The listing builds one solid part. Answer for the finished solid, in the listing's coordinates (mm). Face numbers are marked on the shaded views. A direction names the side the tool comes from. Round coordinates to 2 decimals unless told otherwise and drop trailing zeros. Loops run counter-clockwise (first coordinate to the right, second up) from the corner with the lowest first, then second, coordinate; pieces in that order, holes last. Notation, with made-up numbers: (-27.5, -17) - (-11.5, -17) arc R7 ccw to (-11.5, -7) - close; hole circle Ø4 at (40.25, 38.5). An arc over 180 degrees is marked (long way). One line per item, written item: value.
Autodesk Inventor part; units mm, degrees
ref_plane "to_body_XY" through (0, 0, 0) normal (0, 0, -1) x (1, 0, 0)
ref_plane "to_body_YZ" through (0, 0, 0) normal (1, 0, 0) x (0, -1, 0)
ref_plane "to_body_ZX" through (0, 0, 0) normal (0, -1, 0) x (0, 0, -1)
sketch "_____1" plane through (0, 0, 0) normal (0, 0, 1) x (1, 0, 0)
  line L0 (50, 0) -> (-50, 0)
  line L1 (-4, 12) -> (-4, 4.5)
  line L2 (-4, 4.5) -> (-3.5, 4)
  line L3 (-3.5, 4) -> (3.5, 4)
  line L4 (3.5, 4) -> (4, 4.5)
  line L5 (4, 4.5) -> (4, 12)
  line L6 (4, 12) -> (3.5, 12.5)
  line L7 (3.5, 12.5) -> (-3.5, 12.5)
  line L8 (-3.5, 12.5) -> (-4, 12)
revolve "Revolution1" add sketch "_____1" angle 180 about axis through (50, 0, 0) along (1, 0, 0)
sketch "_____2" plane through (0, 0, 0) normal (1, 0, 0) x (0, 0, -1)
  line L0 (-0.75, -25) -> (0.75, -25)
  line L1 (0.75, -25) -> (0.75, 25)
  line L2 (0.75, 25) -> (-0.75, 25)
  line L3 (-0.75, 25) -> (-0.75, -25)
extrude "Extrusion1" cut sketch "_____2" along normal mid plane 16
sketch "_____3" plane through (0, 0, 0) normal (1, 0, 0) x (0, 0, -1)
  line L0 (0, 8) -> (-17.5, 8)
  line L1 (-17.5, 8) -> (-17.5, 11)
  line L2 (-17.5, 11) -> (-5, 11)
  line L3 (-5, 11) -> (-5, 9.7)
  line L4 (-5, 9.7) -> (0, 9.7)
  line L5 (0, 9.7) -> (0, 8)
  line L6 (0, 8) -> (-17.5, 8)
revolve "Revolution2" cut sketch "_____3" angle 360 about axis through (0, 8, 0) along (0, 0, -1)
pattern_linear "Rectangular Pattern1" count 2 spacing 16 along (0, -1, 0) of "Revolution2"
sketch "_____5" plane through (0, 0, 0) normal (1, 0, 0) x (0, 0, -1)
  line L0 (-12.5, -0.75) -> (-8.5, -0.75)
  line L1 (-8.5, -0.75) -> (-8.5, 0.75)
  line L2 (-8.5, 0.75) -> (-12.5, 0.75)
  line L3 (-12.5, 0.75) -> (-12.5, -0.75)
extrude "Extrusion2" cut sketch "_____5" along normal mid plane 16
ref_plane "to_body_XY" through (0, 0, 0) normal (0, 0, -1) x (1, 0, 0)
ref_plane "to_body_YZ" through (0, 0, 0) normal (1, 0, 0) x (0, -1, 0)
ref_plane "to_body_ZX" through (0, 0, 0) normal (0, -1, 0) x (0, 0, -1)
ref_plane "to_bolt_1_XY" through (0, 8, 5) normal (0, 0, 1) x (1, 0, 0)
ref_plane "to_bolt_1_YZ" through (0, 8, 5) normal (1, 0, 0) x (0, 1, 0)
ref_plane "to_bolt_1_ZX" through (0, 8, 5) normal (0, 1, 0) x (0, 0, 1)
ref_plane "to_bolt_2_XY" through (0, -8, 5) normal (0, 0, 1) x (1, 0, 0)
ref_plane "to_bolt_2_YZ" through (0, -8, 5) normal (1, 0, 0) x (0, 1, 0)
ref_plane "to_bolt_2_ZX" through (0, -8, 5) normal (0, 1, 0) x (0, 0, 1)
properties part number "C-SCNPAW8-8_1"
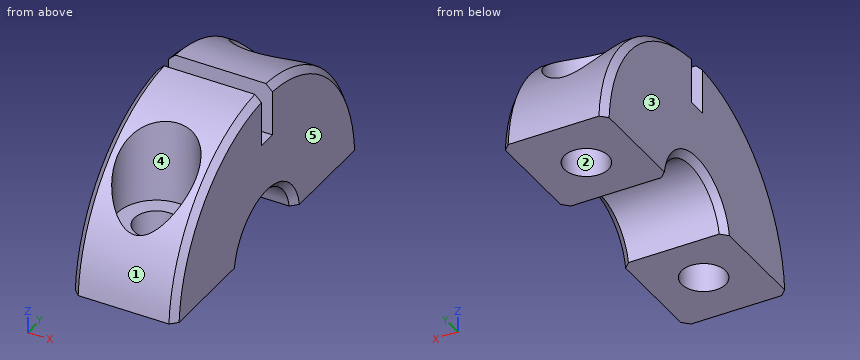
1) A cutting plane is placed at C-C on x = 2.75. Give the vertices of the cut face in (y, z), and give its area (3 significant figures).
Final values:
outline: (-12.48, 0.75) - (-3.93, 0.75) arc R4 cw to (3.93, 0.75) - (12.48, 0.75) arc R12.5 ccw to (9.2, 8.46) - (9.2, 5) - (6.8, 5) - (6.8, 10.49) arc R12.5 ccw to (0.75, 12.48) - (0.75, 8.5) - (-0.75, 8.5) - (-0.75, 12.48) arc R12.5 ccw to (-6.8, 10.49) - (-6.8, 5) - (-9.2, 5) - (-9.2, 8.46) arc R12.5 ccw to start
area: 180 mm2
2) Each of these flat-tipped pins is pushed along its axis until it touches: pin 1 Ø2 at (x, z) = (1, 10) entering from -Y; pin 2 Ø3 at (x, z) = (-1.5, 11) entering from +Y; pin 3 Ø4 at (x, z) = (-2, 7.5) entering from +Y (3 decimals). Where does it stop, or does it pass through?
Final values:
pin 1: y = -5.76
pin 2: y = 7.04
pin 3: y = 11.225
3) Consider L1, parallel to Y at x = 0, z = 9; L2, parallel to X at y = -8, z = 7; L3, parallel to X at y = -8, z = 1.85. Determine where each line is inside the solid, lowest interval first.
Final values:
L1: -5 to -0.75, 0.75 to 5
L2: -4 to -3, 3 to 4
L3: -4 to -1.7, 1.7 to 4
4) For the marked faces 4 and 5, determine the directions among +Z, -Z, +X, -X, +Y, -Y from which every point of the face is accessible in a straight line to the end or side of a thin tool.
Final values:
face 4: +Z
face 5: +Z, -Z, +X, +Y, -Y
5) A cutting plane is placed at A-A on x = 0. Give the vertices of the cut face in (y, z), and give its area (3 significant figures).
Final values:
outline: (-12.48, 0.75) - (-9.7, 0.75) - (-9.7, 5) - (-11, 5) - (-11, 5.94) arc R12.5 ccw to start; (-6.3, 0.75) - (-3.93, 0.75) arc R4 cw to (3.93, 0.75) - (6.3, 0.75) - (6.3, 5) - (5, 5) - (5, 11.46) arc R12.5 ccw to (0.75, 12.48) - (0.75, 8.5) - (-0.75, 8.5) - (-0.75, 12.48) arc R12.5 ccw to (-5, 11.46) - (-5, 5) - (-6.3, 5) - close; (9.7, 0.75) - (12.48, 0.75) arc R12.5 ccw to (11, 5.94) - (11, 5) - (9.7, 5) - close
area: 121 mm2
6) A cutting plane is placed at B-B on z = 2. Give the number of separate pieces and of enclosed holes in the cut face, and give its area (3 significant figures).
Final values:
separate pieces: 2
enclosed holes: 2
area: 123 mm2
7) For a pull along Y with two mould halves and no side action, classify the marked faces 1, 2 and 3 as released by +Y, released by -Y, zero draft, split by the parting line, or undercut.
Final values:
face 1: released by -Y
face 2: undercut
face 3: zero draft
